Read the model definition and answer for the solid it produces. Units are mm, in the model's axes. A direction names the side the tool comes from. Round coordinates to 2 decimals unless told otherwise and drop trailing zeros. Order: outer loops, then holes, each group sorted by start corner. A loop starts at its lowest first (then second) coordinate and runs counter-clockwise, first axis right, second up. Notation, with made-up numbers: (29.25, 2.25) -> (79.25, 2.25) arc R10 ccw to (79.25, 20.25) -> close; hole circle Ø6 at (-34, 79.25). An arc over 180 degrees is marked (long way). Use a Markdown table: item, result. Add a question column.
1. Section C-C, the plane z = 0 is taken. Give the vertices of the cut face in (x, y).
2. For faces 4 (the face through (-37.194, 101.465, -8.259)), 5 (the face through (27, 0, 26)), determine the directions among +Z, -Z, +X, -X, +Y, -Y from which every point of the face is accessible in a straight line to the end or side of a thin tool.
3. Section D-D, the plane y = 178 is taken. Give the vertices of the cut face in (x, z), then the cut area to 3 significant figures.
4. Consider L1, parallel to X at y = 0.5, z = 0; L2, parallel to X at y = 95, z = 1; L3, parallel to Y at x = -30.5, z = 24. Determine where each line is inside the solid, lowest interval first. Write a range as [from, to].
5. The mould has two halves that part along Y. Classify faces 1 (the face through (41.974, 0.902, 1.579)), 2 (the face through (-30.911, 1.252, -40.313)), 3 (the face through (36.21, 179.85, 10.51)): +Y half, -Y half, draft (parallel to the pull), parting line (faces both ways), or undercut.
6. Section B-B, the plane x = -17 is taken. Give the vertices of the cut face in (y, z), then the cut area to 3 significant figures.
7. Section A-A, the plane z = -26 is taken. Give the vertices of the cut face in (x, y), then the cut area to 3 significant figures.
8. Given pin 1 (5 mm diameter, centred on y = 171.5, z = -6.5, fed in from -X); pin 2 (3 mm diameter, centred on y = 61, z = 15.5, fed in from +X); pin 3 (2 mm diameter, centred on x = 28.5, y = 83.5, fed in from -Z); pin 4 (4.5 mm diameter, centred on x = 0, z = 44.45, fed in from -Y), each flat-ended and moving along its own axis, determine where each tip first touches the part or whether it passes through.
```python
from build123d import *

# Parameters (mm, degrees)
SKETCH1_R                                  = 38.1
SKETCH1_R_2                                = 36.83
BOSS_EXTRUDE1_DEPTH                        = 203.2
SKETCH2_R                                  = 12.7
CUT_EXTRUDE1_DEPTH                         = 211.222406037
CIRPATTERN2_COUNT                          = 2
CIRPATTERN2_ANGLE                          = 80
SKETCH5_R                                  = 50.8
SKETCH5_R_2                                = 38.1
BOSS_EXTRUDE2_DEPTH                        = 2.54
CSK_FOR_10_FLAT_HEAD_MACHINE_SCREW_2_COUNT = 2
CSK_FOR_10_FLAT_HEAD_MACHINE_SCREW_2_PITCH = 62.861792847
CIRPATTERN3_COUNT                          = 2


with BuildPart() as part:
    # Sketch1 → Boss-Extrude1 (new body)
    with BuildSketch(Plane(origin=(0, 0, 0), x_dir=(1, 0, 0), z_dir=(0, 1, 0))):
        with Locations(Location((0, 0, 0), (0, 0, 270))):
            Circle(SKETCH1_R)
        with Locations(Location((0, 0, 0), (0, 0, 270))):
            Circle(SKETCH1_R_2, mode=Mode.SUBTRACT)
    extrude(amount=BOSS_EXTRUDE1_DEPTH)

    # Sketch2 → Cut-Extrude1 (cut, through all)
    with BuildSketch(Plane(origin=(0, 0, 0), x_dir=(0, 0, -1), z_dir=(1, 0, 0))):
        with Locations(Location((0, 172.72, 0), (0, 0, 180))):
            Circle(SKETCH2_R)
    cut_extrude1 = extrude(amount=CUT_EXTRUDE1_DEPTH, mode=Mode.SUBTRACT)

    # CirPattern2: Cut-Extrude1 ×2 about axis
    cirpattern2_axis = Axis((0, 203.2, 0), (0, -1, 0))
    for i in range(1, CIRPATTERN2_COUNT):
        add(cut_extrude1.rotate(cirpattern2_axis, i * CIRPATTERN2_ANGLE / (CIRPATTERN2_COUNT - 1)), mode=Mode.SUBTRACT)

    # Sketch5 → Boss-Extrude2 (add)
    with BuildSketch(Plane(origin=(0, 0, 0), x_dir=(1, 0, 0), z_dir=(0, 1, 0))):
        with Locations(Location((0, 0, 0), (0, 0, 270))):
            Circle(SKETCH5_R)
        with Locations(Location((0, 0, 0), (0, 0, 270))):
            Circle(SKETCH5_R_2, mode=Mode.SUBTRACT)
    extrude(amount=BOSS_EXTRUDE2_DEPTH)

    # Sketch7 → CSK for #10 Flat Head Machine Screw (100)1 (revolve, cut)
    with BuildSketch(Plane(origin=(0, 2.54, -44.45), x_dir=(0, 0, 1), z_dir=(1, 0, 0))):
        Polygon((0, 0), (0, 2.54), (2.8067, 2.54), (2.8067, 1.747676712), (4.8895, 0), align=None)
    csk_for_10_flat_head_machine_screw_100 = revolve(axis=Axis((0, 8.89, -44.45), (0, -1, 0)), mode=Mode.SUBTRACT)

    # CSK for _10 Flat Head Machine Screw  2: CSK for #10 Flat Head Machine Screw (100)1 ×2
    with Locations(*[Vector(0.7071067811865476, 0, 0.7071067811865476) * (i * CSK_FOR_10_FLAT_HEAD_MACHINE_SCREW_2_PITCH) for i in range(1, CSK_FOR_10_FLAT_HEAD_MACHINE_SCREW_2_COUNT)]):
        add(csk_for_10_flat_head_machine_screw_100, mode=Mode.SUBTRACT)

    # CirPattern3: CSK for #10 Flat Head Machine Screw (100)1 ×2 about axis
    cirpattern3_axis = Axis((0, 0, 0), (0, 1, 0))
    for i in range(1, CIRPATTERN3_COUNT):
        add(csk_for_10_flat_head_machine_screw_100.rotate(cirpattern3_axis, i * 360 / CIRPATTERN3_COUNT), mode=Mode.SUBTRACT)

    # CirPattern3 copy 1 sketch → CirPattern3 copy 1 (revolve, cut)
    with BuildSketch(Plane(origin=(-44.45, 2.54, 0), x_dir=(0, 0, -1), z_dir=(-1, 0, 0))):
        Polygon((0, 0), (0, 2.54), (2.8067, 2.54), (2.8067, 1.747676712), (4.8895, 0), align=None)
    revolve(axis=Axis((-44.45, 8.89, 0), (0, -1, 0)), mode=Mode.SUBTRACT)


solid = part.part
```
Verdict:
| question | item | result |
|---|---|---|
| 1 | outline | (-50.8, 0) -> (-47.26, 0) -> (-47.26, 0.79) -> (-49.34, 2.54) -> (-50.8, 2.54) -> close; (-41.64, 0) -> (-36.83, 0) -> (-36.83, 203.2) -> (-38.1, 203.2) -> (-38.1, 2.54) -> (-39.56, 2.54) -> (-41.64, 0.79) -> close; (36.83, 0) -> (41.64, 0) -> (41.64, 0.79) -> (39.56, 2.54) -> (38.1, 2.54) -> (38.1, 160.02) -> (36.83, 160.02) -> close; (36.83, 185.42) -> (38.1, 185.42) -> (38.1, 203.2) -> (36.83, 203.2) -> close; (47.26, 0) -> (50.8, 0) -> (50.8, 2.54) -> (49.34, 2.54) -> (47.26, 0.79) -> close |
| 2 | face 4 | +Y |
| 2 | face 5 | +Z, -Z, +X, -X, -Y |
| 3 | outline | (-5.3, 36.45) -> (-5.07, 37.76) arc R38.1 ccw (long way) to (36.31, -11.55) -> (34.97, -11.55) arc R36.83 cw (long way) to start; (17.45, 32.43) arc R36.83 cw to (34.97, 11.55) -> (36.31, 11.55) arc R38.1 ccw to (17.68, 33.75) -> close |
| 3 | area | 239 mm2 |
| 4 | L1 | x = [-50.8, -47.26], [-41.64, -36.83], [36.83, 41.64], [47.26, 50.8] |
| 4 | L2 | x = [-38.09, -36.82], [36.82, 38.09] |
| 4 | L3 | y = [0, 2.54] |
| 5 | face 1 | +Y half |
| 5 | face 2 | draft |
| 5 | face 3 | undercut |
| 6 | outline | (0, -47.87) -> (2.54, -47.87) -> (2.54, -34.1) -> (203.2, -34.1) -> (203.2, -32.67) -> (0, -32.67) -> close; (0, 32.67) -> (203.2, 32.67) -> (203.2, 34.1) -> (2.54, 34.1) -> (2.54, 47.87) -> (0, 47.87) -> close |
| 6 | area | 649 mm2 |
| 7 | outline | (-43.64, 0) -> (-26.09, 0) -> (-26.09, 203.2) -> (-27.85, 203.2) -> (-27.85, 2.54) -> (-43.64, 2.54) -> close; (26.09, 0) -> (43.64, 0) -> (43.64, 2.54) -> (27.85, 2.54) -> (27.85, 203.2) -> (26.09, 203.2) -> close |
| 7 | area | 797 mm2 |
| 8 | pin 1 | stops at x = -37.89 |
| 8 | pin 2 | stops at x = 35.43 |
| 8 | pin 3 | stops at z = -26.37 |
| 8 | pin 4 | passes through |
